The model under review builds one solid part; all positions refer to its coordinate system, in mm. Face numbers are marked on the shaded views. Give positions to 0.01 mm unless a question says otherwise; leave off trailing zeros. Order: outer loops, then holes, each group sorted by start corner. A loop starts at its lowest first (then second) coordinate and runs counter-clockwise, first axis right, second up. Notation, with made-up numbers: (-40, 47) - (-28, 47) arc R28 ccw to (-28, 66) - close; hole circle Ø9 at (28.25, 30). An arc over 180 degrees is marked (long way). Use CSV: the item, a comma, the result in double quotes. Start each with the question number.
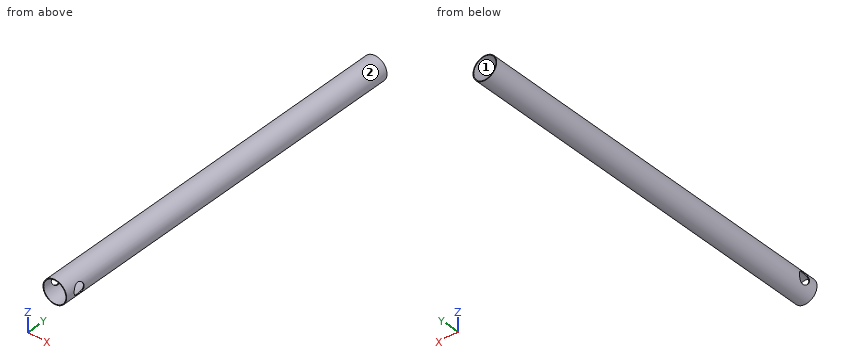
```python
from build123d import *

# Parameters (mm, degrees)
SKETCH1_R           = 25.4
BOSS_EXTRUDE1_DEPTH = 406.4
SHELL1_T            = -1.5875
SKETCH2_R           = 12.7
CUT_EXTRUDE1_DEPTH  = 411.349558304


with BuildPart() as part:
    # Sketch1 → Boss-Extrude1 (new, symmetric)
    with BuildSketch(Plane(origin=(0, 0, 0), x_dir=(1, 0, 0), z_dir=(0, 1, 0))):
        with Locations(Location((0, 0, 0), (0, 0, 270))):
            Circle(SKETCH1_R)
    extrude(amount=BOSS_EXTRUDE1_DEPTH, both=True)

    # Shell1
    shell1_openings = [part.faces().sort_by_distance(p)[0] for p in [
        (0, 406.4, 0),
        (0, -406.4, 0),
    ]]
    offset(amount=SHELL1_T, openings=shell1_openings, kind=Kind.INTERSECTION)

    # Sketch2 → Cut-Extrude1 (cut, through all)
    with BuildSketch(Plane(origin=(25.4, 0, 0), x_dir=(0, 0, -1), z_dir=(1, 0, 0))):
        with Locations((0, -374.65)):
            Circle(SKETCH2_R)
    extrude(amount=-CUT_EXTRUDE1_DEPTH, mode=Mode.SUBTRACT)


solid = part.part
```
1. Mouldability with a two-part tool opening along Z and no side actions: class the marked faces 1 and 2 as pulls with the +Z half, pulls with the -Z half, needs draft (parallel to the pull), parting line crosses it, or undercut.
2. Consider section C-C (y = -374.65). Give the boundary of the cut face in (x, z) (1 decimal), and give its area (3 significant figures).
3. Clearance check with flat-ended pins moving along their axes: pin 1 (1.5 mm diameter, centred on y = 155, z = -14.5, fed in from +X); pin 2 (8 mm diameter, centred on y = -223.5, z = 6.5, fed in from +X); pin 3 (12 mm diameter, centred on x = -7, y = 2, fed in from +Z). State where each tip first meets the part, or that it passes through.
4. Consider section B-B (z = 0). Give the boundary of the cut face in (x, y).
5. To check wall thickness, follow L1, parallel to X at y = 234, z = 0; L2, parallel to X at y = 89, z = -2; L3, parallel to Y at x = -24.2, z = 0. State the ranges of each line that lie inside material, in increasing order. Write a range as [from, to].
6. Consider section A-A (x = 0). Give the boundary of the cut face in (y, z).
Answers follow:
1,face 1,"undercut"
1,face 2,"parting line crosses it"
2,outline,"(-22, -12.7) arc R25.4 ccw to (22, -12.7) - (20.1, -12.7) arc R23.8 cw to (-20.1, -12.7) - close; (-22, 12.7) - (-20.1, 12.7) arc R23.8 cw to (20.1, 12.7) - (22, 12.7) arc R25.4 ccw to start"
2,area,"161 mm^2"
3,pin 1,"stops at x = 21.36"
3,pin 2,"stops at x = 25.28"
3,pin 3,"stops at z = 25.38"
4,outline,"(-25.4, -406.4) - (-23.81, -406.4) - (-23.81, -387.35) - (-25.4, -387.35) - close; (-25.4, -361.95) - (-23.81, -361.95) - (-23.81, 406.4) - (-25.4, 406.4) - close; (23.81, -406.4) - (25.4, -406.4) - (25.4, -387.35) - (23.81, -387.35) - close; (23.81, -361.95) - (25.4, -361.95) - (25.4, 406.4) - (23.81, 406.4) - close"
5,L1,"x = [-25.4, -23.81], [23.81, 25.4]"
5,L2,"x = [-25.32, -23.73], [23.73, 25.32]"
5,L3,"y = [-406.4, -387.35], [-361.95, 406.4]"
6,outline,"(-406.4, -25.4) - (406.4, -25.4) - (406.4, -23.81) - (-406.4, -23.81) - close; (-406.4, 23.81) - (406.4, 23.81) - (406.4, 25.4) - (-406.4, 25.4) - close"
